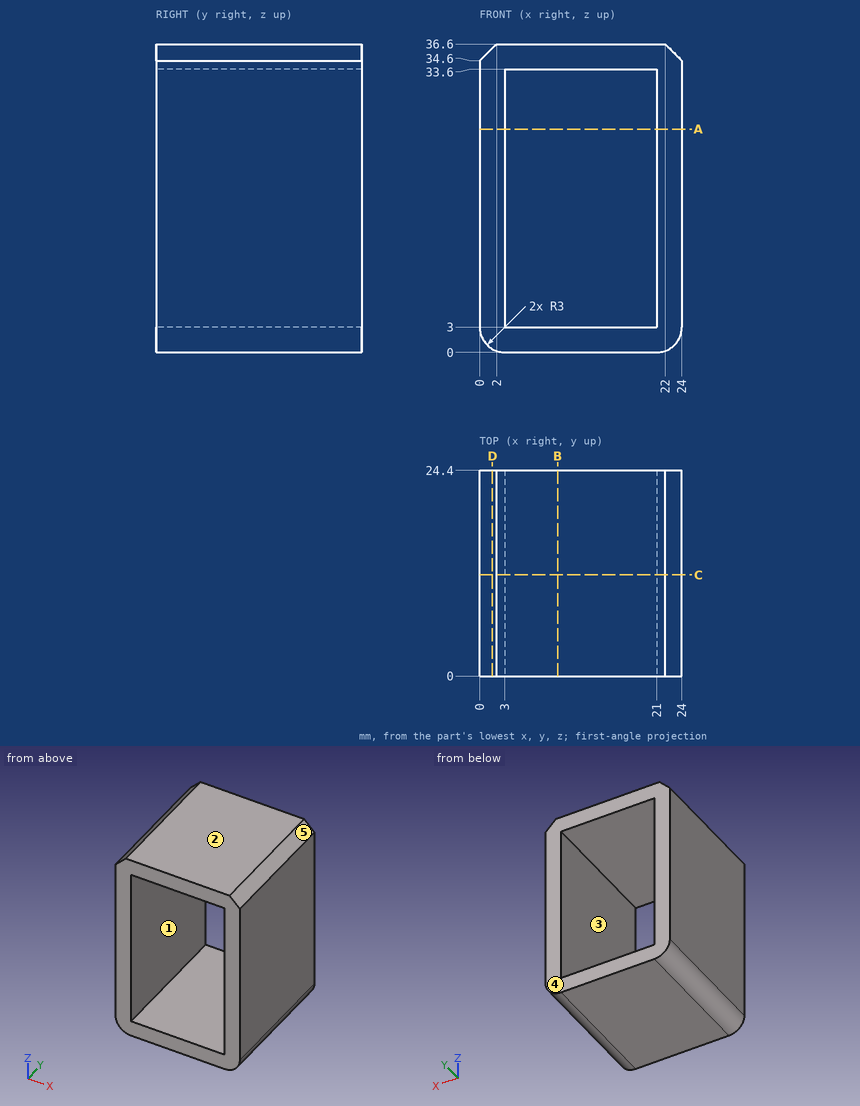
The drawing under review shows one solid part. Ordinate dimensions are in mm from its lowest x, y, z. A direction names the side the tool comes from. Round coordinates to 2 decimals unless told otherwise and drop trailing zeros. Order: outer loops, then holes, each group sorted by start corner. A loop starts at its lowest first (then second) coordinate and runs counter-clockwise, first axis right, second up. Notation, with made-up numbers: (-34.75, 86) -> (-2.75, 86) arc R24 ccw to (-2.75, 106) -> close; hole circle Ø9 at (84, 72.25). An arc over 180 degrees is marked (long way). Use a Markdown table: item, result.
Item 1: Take a section at A-A (z = 26.5). State the section outline as (x, y) points.
Resolved:
| item | result |
|---|---|
| outline | (0, 0) -> (3, 0) -> (3, 24.4) -> (0, 24.4) -> close; (21, 0) -> (24, 0) -> (24, 24.4) -> (21, 24.4) -> close |
Item 2: Draft analysis for pull direction Z (two halves, no side actions). For the marked faces 3, 4 and 5, state which applies: +Z half, -Z half, draft (parallel to the pull), parting line (faces both ways), or undercut.
Resolved:
| item | result |
|---|---|
| face 3 | undercut |
| face 4 | draft |
| face 5 | +Z half |
Item 3: Take a section at B-B (x = 9.25). State the section outline as (y, z) points, plus the area to 3 significant figures.
Resolved:
| item | result |
|---|---|
| outline | (0, 0) -> (24.4, 0) -> (24.4, 3) -> (0, 3) -> close; (0, 33.6) -> (24.4, 33.6) -> (24.4, 36.6) -> (0, 36.6) -> close |
| area | 146 mm² |
Item 4: Machinability: for the marked faces 1 and 2, which of the approach directions +Z, -Z, +X, -X, +Y, -Y give a long, thin tool a straight path to every point of the face, cutting with its end or side? Answer none if there is none.
Resolved:
| item | result |
|---|---|
| face 1 | +Y, -Y |
| face 2 | +Z, +X, -X, +Y, -Y |
Item 5: Take a section at C-C (y = 12). State the section outline as (x, z) points, plus the area to 3 significant figures.
Resolved:
| item | result |
|---|---|
| outline | (0, 3) arc R3 ccw to (3, 0) -> (21, 0) arc R3 ccw to (24, 3) -> (24, 34.6) -> (22, 36.6) -> (2, 36.6) -> (0, 34.6) -> close; hole (3, 3) -> (21, 3) -> (21, 33.6) -> (3, 33.6) -> close |
| area | 320 mm² |
Item 6: For line 1 along Z through (x, y) = (3.75, 12); line 2 along X through (y, z) = (11.5, 7.5); line 3 along Z through (x, y) = (23.25, 1.5), list the stretches that pass through material, from the lowest coordinate up. Write a range as [from, to].
Resolved:
| item | result |
|---|---|
| line 1 | z = [0, 3], [33.6, 36.6] |
| line 2 | x = [0, 3], [21, 24] |
| line 3 | z = [1.02, 35.35] |
Item 7: Take a section at D-D (x = 1.5). State the section outline as (y, z) points, plus the area to 3 significant figures.
Resolved:
| item | result |
|---|---|
| outline | (0, 0.4) -> (24.4, 0.4) -> (24.4, 36.1) -> (0, 36.1) -> close |
| area | 871 mm² |
